Can you work these out from the model? Positions are in its coordinate system, mm. Face numbers are marked on the shaded views. A direction names the side the tool comes from. Round coordinates to 2 decimals unless told otherwise and drop trailing zeros. Order: outer loops, then holes, each group sorted by start corner. A loop starts at its lowest first (then second) coordinate and runs counter-clockwise, first axis right, second up. Notation, with made-up numbers: (-20, 78) -> (23, 78) arc R20 cw to (23, 116) -> close; hole circle Ø4 at (-15.75, 21). An arc over 180 degrees is marked (long way). Use a Markdown table: item, result. Add a question column.
Q1. If we section it at B-B on y = 2.75: List the corners of the cut face in (x, z) for me (3 decimals).
Q2. We'd pull the mould along Z, two halves only. Please class the marked faces 3, 4, 5 and 6: +Z half, -Z half, draft (parallel to the pull), parting line (faces both ways), or undercut.
Q3. If we section it at A-A on x = 8.5: List the corners of the cut face in (y, z) for me (3 decimals).
Q4. For the marked faces 1 and 2, which set-ups out of +Z, -Z, +X, -X, +Y, -Y let a thin tool reach every point of the face, with its end or its side?
Q5. I need wall thicknesses on line 1 along Y through (x, z) = (0.5, -6) (3 decimals); line 2 along Y through (x, z) = (9, -11) (3 decimals); line 3 along Y through (x, z) = (1.75, -5) (3 decimals). Which ranges of each line are inside material? Lowest first, please. Write a range as [from, to].
Q6. If we section it at C-C on x = 3: Give the number of separate pieces and of enclosed holes in the cut face, plus the area to 3 significant figures.
Q7. If we section it at D-D on z = 0.25: List the corners of the cut face in (x, y) for me (3 decimals).
Q8. I'm going to push flat-ended pins straight in: pin 1 Ø1.5 at (x, z) = (2.5, -12.5) entering from +Y; pin 2 Ø1 at (y, z) = (10, -9.5) entering from +X; pin 3 Ø4 at (y, z) = (13.125, -6.125) entering from -X; pin 4 Ø4 at (x, z) = (8.5, -10) entering from +Y (3 decimals). Where does each tip first touch, or does it pass through?
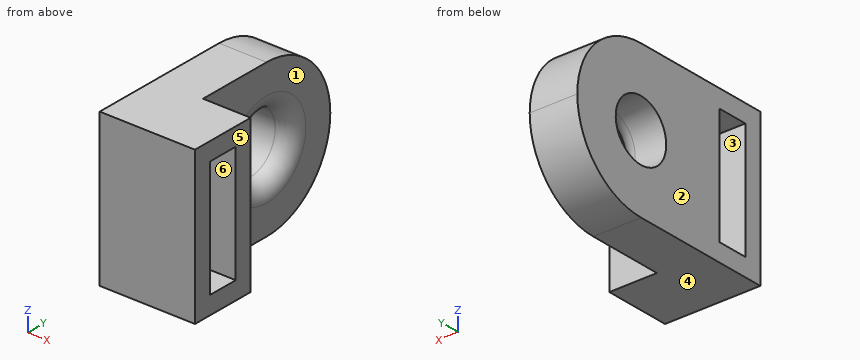
Autodesk Inventor part; units mm, degrees
ref_plane "YZ Plane" through (0, 0, 0) normal (1, 0, 0) x (0, 1, 0)
ref_plane "XZ Plane" through (0, 0, 0) normal (0, 1, 0) x (-1, 0, 0)
ref_plane "XY Plane" through (0, 0, 0) normal (0, 0, 1) x (1, 0, 0)
sketch "Sketch1" plane through (0, 0, 0) normal (1, 0, 0) x (0, 1, 0)
  line L0 (0, 0) -> (3.25, 0)
  line L1 (3.25, 0) -> (3.25, -12.25)
  line L2 (3.25, -12.25) -> (0, -12.25)
  line L3 (0, -12.25) -> (0, 0)
  line L4 (-1.875, -14.125) -> (5.125, -14.125)
  line L5 (5.125, -14.125) -> (5.125, 1.875)
  line L6 (5.125, 1.875) -> (-1.875, 1.875)
  line L7 (-1.875, 1.875) -> (-1.875, -14.125)
  line L8 (-1.875, -14.125) -> (5.125, 1.875) construction
  line L9 (5.125, -14.125) -> (-1.875, 1.875) construction
  point P0 (1.625, -6.125)
  dimension "d0" = 3.25
  dimension "d1" = 12.25
  dimension "d2" = 7
  dimension "d3" = 16
extrude "Extrusion1" add sketch "Sketch1" along normal blind 10
sketch "Sketch2" plane through (0, 5.125, 1.875) normal (0, 1, 0) x (1, 0, 0)
  line L0 (0, 0) -> (0, 16)
  line L1 (0, 16) -> (10, 16)
  line L2 (0, 0) -> (5, 0)
  line L3 (5, 0) -> (5, 16)
  line L4 (5, 16) -> (0, 16)
  line L5 (0, 16) -> (0, 0)
  point P0 (0, 1.875)
  dimension "d6" = 5
extrude "Extrusion2" add sketch "Sketch2" along normal blind 16
sketch "Sketch3" plane through (5, 5.125, 1.875) normal (1, 0, 0) x (0, 0, -1)
  line L0 (16, 0) -> (0, 0) construction
  line L1 (0, -7) -> (0, 16) construction
  line L2 (16, 0) -> (0, 16) construction
  circle A0 centre (8, 8) radius 3.175
  point P0 (1.875, -5.125)
  dimension "d9" = 6.35
extrude "Extrusion3" cut sketch "Sketch3" against normal blind 16
fillet "Fillet1" radius 8 2 edges at (2.5, 21.125, 1.875) (2.5, 21.125, -14.125)
fillet "Fillet2" radius 1.75 1 edges at (5, 13.125, -2.95)
properties part number "frameAdjustment 11-28"
Answer below:
| question | item | result |
|---|---|---|
| 1 | outline | (0, -14.125) -> (10, -14.125) -> (10, -12.25) -> (0, -12.25) -> close; (0, 0) -> (10, 0) -> (10, 1.875) -> (0, 1.875) -> close |
| 2 | face 3 | undercut |
| 2 | face 4 | -Z half |
| 2 | face 5 | draft |
| 2 | face 6 | undercut |
| 3 | outline | (-1.875, -14.125) -> (5.125, -14.125) -> (5.125, 1.875) -> (-1.875, 1.875) -> close; hole (0, -12.25) -> (3.25, -12.25) -> (3.25, 0) -> (0, 0) -> close |
| 4 | face 1 | +Z, -Z, +X, +Y |
| 4 | face 2 | +Z, -Z, -X, +Y, -Y |
| 5 | line 1 | [-1.875, 0], [3.25, 9.952], [16.298, 21.124] |
| 5 | line 2 | [-1.875, 0], [3.25, 5.125] |
| 5 | line 3 | [-1.875, 0], [3.25, 10.156], [16.094, 21.046] |
| 6 | separate pieces | 1 |
| 6 | enclosed holes | 2 |
| 6 | area | 269 mm² |
| 7 | outline | (0, -1.875) -> (10, -1.875) -> (10, 5.125) -> (5, 5.125) -> (5, 17.958) -> (0, 17.958) -> close |
| 8 | pin 1 | y = 18.81 |
| 8 | pin 2 | x = 5 |
| 8 | pin 3 | through |
| 8 | pin 4 | y = 5.125 |
